Can you work these out from the model? Positions are in its coordinate system, mm. Face numbers are marked on the shaded views. A direction names the side the tool comes from. Give positions to 0.01 mm unless a question says otherwise; leave off trailing zeros. Order: outer loops, then holes, each group sorted by start corner. A loop starts at its lowest first (then second) coordinate and runs counter-clockwise, first axis right, second up. Notation, with made-up numbers: (14.25, 50.5) - (44.25, 50.5) arc R30 ccw to (44.25, 83.5) - close; hole circle Ø3 at (-22.75, 3). An arc over 180 degrees is marked (long way). Return JSON: item names as keys, results as strings.
```python
from build123d import *

# Parameters (mm, degrees)
SKETCH_2_R          = 2.5
CUT_EXTRUDE_1_DEPTH = 55
SKETCH_3_R          = 6
CUT_EXTRUDE_2_DEPTH = 5
CUT_EXTRUDE_START   = -5
SKETCH_4_R          = 6
CUT_EXTRUDE_3_DEPTH = 5


with BuildPart() as part:
    # 草图1 → 旋转1 (revolve)
    with BuildSketch(Plane(origin=(0, 0, 0), x_dir=(1, 0, 0), z_dir=(0, 1, 0)), mode=Mode.PRIVATE) as revolve_1_sk:
        with BuildLine():
            Line((-6.5, 6.5), (-6.5, -6.5))
            Line((-6.5, -6.5), (6.5, -6.5))
            Line((6.5, -6.5), (6.5, 6.5))
            Line((6.5, 6.5), (5.477225575, 6.5))
            ThreePointArc((5.477225575, 6.5), (0, 3.5), (-5.477225575, 6.5))
            Line((-5.477225575, 6.5), (-6.5, 6.5))
        make_face()
    revolve(revolve_1_sk.sketch.rotate(Axis((-6.5, 0, 6.5), (1, 0, 0)), 180), axis=Axis((-6.5, 0, 6.5), (1, 0, 0)))

    # 草图2 → 切除-拉伸1 (cut)
    with BuildSketch(Plane(origin=(6.5, 0, 0), x_dir=(0, 0, -1), z_dir=(1, 0, 0))):
        with Locations((-6.5, 0)):
            Circle(SKETCH_2_R)
    extrude(amount=-CUT_EXTRUDE_1_DEPTH, mode=Mode.SUBTRACT)

    # 草图3 → 切除-拉伸2 (cut)
    with BuildSketch(Plane(origin=(6.5, 0, 0), x_dir=(0, 0, -1), z_dir=(1, 0, 0))):
        with Locations((-6.5, 0)):
            Circle(SKETCH_3_R)
    extrude(amount=-CUT_EXTRUDE_2_DEPTH, mode=Mode.SUBTRACT)

    # 草图4 → 切除-拉伸3 (cut)
    with BuildSketch(Plane.ZY.offset(6.5).offset(CUT_EXTRUDE_START)):
        with Locations(Location((6.5, 0, 0), (0, 0, 180))):
            Circle(SKETCH_4_R)
    extrude(amount=CUT_EXTRUDE_3_DEPTH, mode=Mode.SUBTRACT)


solid = part.part
```
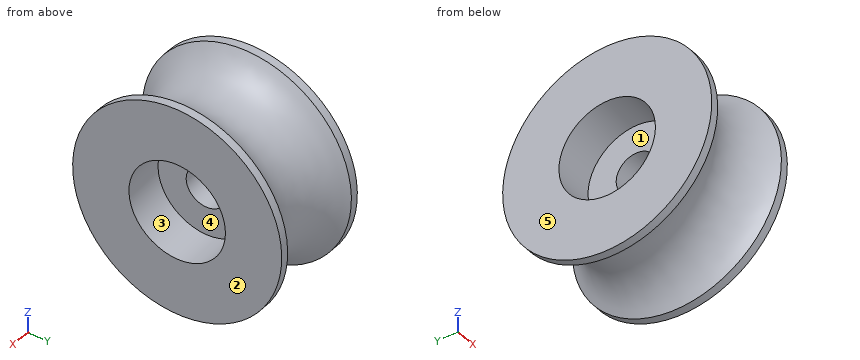
1. If I drill on L1, parallel to X at y = -11, z = 0.25; L2, parallel to X at y = -8.5, z = 16; L3, parallel to Z at x = 2.25, y = -8.5, over which ranges is the centre line in solid material (lowest first)? Write a range as [from, to].
Checks:
{"L1": "[-6.5, -5.24], [5.24, 6.5]", "L2": "[-6.5, -5.31], [5.31, 6.5]", "L3": "[0.5, 12.5]"}
2. Suppose I cut it at C-C (x = 0). List the corners of the cut face in (y, z) for me.
Checks:
{"outline": "circle Ø20 at (0, 6.5); hole circle Ø5 at (0, 6.5)"}
3. For pin 1 Ø6 at (x, z) = (1.5, 0.5) entering from -Y; pin 2 Ø3.5 at (y, z) = (-1, 7) entering from -X; pin 3 Ø11 at (y, z) = (0, 6.5) entering from +X, each with a flat end and sliding along its axis, tell me the tip position at first contact or that it passes through.
Checks:
{"pin 1": "y = -10.54", "pin 2": "x = -1.5", "pin 3": "x = 1.5"}
4. Suppose I cut it at B-B (y = 0). List the corners of the cut face in (x, z) for me.
Checks:
{"outline": "(-6.5, -6.5) - (-5.48, -6.5) arc R6.5 cw to (5.48, -6.5) - (6.5, -6.5) - (6.5, 0.5) - (1.5, 0.5) - (1.5, 4) - (-1.5, 4) - (-1.5, 0.5) - (-6.5, 0.5) - close; (-6.5, 12.5) - (-1.5, 12.5) - (-1.5, 9) - (1.5, 9) - (1.5, 12.5) - (6.5, 12.5) - (6.5, 19.5) - (5.48, 19.5) arc R6.5 cw to (-5.48, 19.5) - (-6.5, 19.5) - close"}
5. Suppose I cut it at D-D (x = -2). List the corners of the cut face in (y, z) for me.
Checks:
{"outline": "circle Ø20.63 at (0, 6.5); hole circle Ø12 at (0, 6.5)"}
6. Suppose I cut it at A-A (z = 6.5). List the corners of the cut face in (x, y) for me, plus the area to 3 significant figures.
Checks:
{"outline": "(-6.5, -13) - (-5.48, -13) arc R6.5 cw to (5.48, -13) - (6.5, -13) - (6.5, -6) - (1.5, -6) - (1.5, -2.5) - (-1.5, -2.5) - (-1.5, -6) - (-6.5, -6) - close; (-6.5, 6) - (-1.5, 6) - (-1.5, 2.5) - (1.5, 2.5) - (1.5, 6) - (6.5, 6) - (6.5, 13) - (5.48, 13) arc R6.5 cw to (-5.48, 13) - (-6.5, 13) - close", "area": "157 mm^2"}
7. On a 3-axis mill with a long thin cutter (end or side, diameter ignored), from which of +Z, -Z, +X, -X, +Y, -Y can I reach the whole of each face in a straight line? I mean the marked faces 1, 2 and 3. Say none if no direction works.
Checks:
{"face 1": "-X", "face 2": "+Z, -Z, +X, +Y, -Y", "face 3": "+X"}
8. Thinking about a two-plate mould opening in Y: for the marked faces 4 and 5, which applies, +Y half, -Y half, draft (parallel to the pull), parting line (faces both ways), or undercut?
Checks:
{"face 4": "undercut", "face 5": "draft"}
